```python
from build123d import *

# Parameters (mm, degrees)
F1_DEPTH  = 35
F2_R      = 30
F5_DEPTH  = 3
F8_DEPTH  = 3
F10_DEPTH = 2
F11_R     = 1.999


# Not quite as in the source:
# - a fillet or chamfer is up to 0.001 mm smaller than in the source, because OpenCascade refuses the exact size


with BuildPart() as f1:
    # F0 (on Right) → F1 (new body, symmetric)
    with BuildSketch(Plane.YZ):
        with BuildLine():
            Line((-75, 163), (-78, 163))
            Line((-78, 163), (-78, 8))
            ThreePointArc((-78, 8), (-75.6568542495, 2.3431457505), (-70, 0))
            Line((-70, 0), (0, 0))
            Line((0, 0), (0, 3))
            Line((0, 3), (-67, 3))
            ThreePointArc((-67, 3), (-72.6568542495, 5.3431457505), (-75, 11))
            Line((-75, 11), (-75, 163))
        make_face()
        with BuildLine():
            Line((0, 3), (0, 0))
            Line((0, 0), (70, 0))
            ThreePointArc((70, 0), (75.6568542495, 2.3431457505), (78, 8))
            Line((78, 8), (78, 163))
            Line((78, 163), (75, 163))
            Line((75, 163), (75, 11))
            ThreePointArc((75, 11), (72.6568542495, 5.3431457505), (67, 3))
            Line((67, 3), (0, 3))
        make_face()
    extrude(amount=F1_DEPTH, both=True)

    # F2
    f2_edges = [f1.edges().sort_by_distance(p)[0] for p in [
        (35, -76.5, 163),
        (35, 76.5, 163),
        (-35, 76.5, 163),
        (-35, -76.5, 163),
    ]]
    fillet(f2_edges, radius=F2_R)

    # F4 (on offset) → F5 (join)
    with BuildSketch(Plane(origin=(-35, 0, 0), x_dir=(0, -1, 0), z_dir=(-1, 0, 0))):
        with BuildLine():
            Line((-75, 133), (-78, 133))
            Line((-78, 133), (-78, 8))
            ThreePointArc((-78, 8), (-75.6568542495, 2.3431457505), (-70, 0))
            Line((-70, 0), (0, 0))
            Line((0, 0), (70, 0))
            ThreePointArc((70, 0), (75.6568542495, 2.3431457505), (78, 8))
            Line((78, 8), (78, 133))
            Line((78, 133), (75, 133))
            Line((75, 133), (0, 123))
            Line((0, 123), (-75, 133))
        make_face()
    extrude(amount=-F5_DEPTH)

    # F7 (on offset) → F8 (join)
    with BuildSketch(Plane.YZ.offset(35)):
        with BuildLine():
            Line((-78, 145), (-78, 8))
            ThreePointArc((-78, 8), (-75.6568542495, 2.3431457505), (-70, 0))
            Line((-70, 0), (0, 0))
            Line((0, 0), (70, 0))
            ThreePointArc((70, 0), (75.6568542495, 2.3431457505), (78, 8))
            Line((78, 8), (78, 145))
            Line((78, 145), (0, 145))
            Line((0, 145), (-78, 145))
        make_face()
    extrude(amount=-F8_DEPTH)

    # F9 (on offset) → F10 (join)
    with BuildSketch(Plane(origin=(-35, 0, 0), x_dir=(0, -1, 0), z_dir=(-1, 0, 0))):
        with BuildLine():
            add(Edge.make_bspline(
                [(22.5, 95), (22.5, 116.6506350946), (-11.25, 105.8253175473), (-45, 95), (-11.25, 84.1746824527), (22.5, 73.3493649054), (22.5, 95)],
                knots=[0, 0, 0, 2.0943951024, 2.0943951024, 4.1887902048, 4.1887902048, 6.2831853072, 6.2831853072, 6.2831853072], degree=2, weights=[1, 0.5, 1, 0.5, 1, 0.5, 1]))
        make_face()
    extrude(amount=F10_DEPTH)

    # F11 (radius 2 in the source; OpenCascade refuses exactly that, so slightly less here)
    f11_edges = [f1.edges().sort_by_distance(p)[0] for p in [
        (-37, 22.5, 95.000001),
    ]]
    fillet(f11_edges, radius=F11_R)


solid = f1.part
```
Can you work these out from the model? Positions are in its coordinate system, mm. A direction names the side the tool comes from. Coordinates: 2 decimals unless noted, no trailing zeros. Order: outer loops, then holes, each group sorted by start corner. A loop starts at its lowest first (then second) coordinate and runs counter-clockwise, first axis right, second up. Notation, with made-up numbers: (37, 52.25) -> (50, 52.25) arc R32 cw to (50, 90.25) -> close; hole circle Ø1 at (70.5, 87). An arc over 180 degrees is marked (long way). Write each question's results on one line, items separated by ' | '.
Item 1: I'm going to push flat-ended pins straight in: pin 1 Ø6 at (x, y) = (1, -48) entering from +Z; pin 2 Ø0.9 at (x, y) = (34, -11) entering from +Z. Where does each tip first touch, or does it pass through?
Results are:
pin 1: z = 3 | pin 2: z = 145
Item 2: I want a section at B-B, the plane y = -57. Write out the boundary of the cut face in (x, z).
Results are:
outline: (-35, 0) -> (35, 0) -> (35, 145) -> (32, 145) -> (32, 3) -> (-32, 3) -> (-32, 130.6) -> (-35, 130.6) -> close
Item 3: Which directions (+Z, -Z, +X, -X, +Y, -Y) give clear straight access to the entire face, cutting with the end or side of a thin tool? Please do faces 5 (the face through (-32, 1, 69)), 6 (the face through (-33.52, -38.02, 128.07)), 7 (the face through (21.23, 76.48, 158.23)).
Results are:
face 5: +Z | face 6: +Z, -X | face 7: +Z, +X, +Y, -Y
Item 4: If I drill on line 1 along X through (y, z) = (-27.5, 76); line 2 along Y through (x, z) = (-8, 67); line 3 along Z through (x, y) = (-26.5, 45.5), over which ranges is the centre line in solid material (lowest first)?
Results are:
line 1: -35 to -32, 32 to 35 | line 2: -78 to -75, 75 to 78 | line 3: 0 to 3
Item 5: I want a section at C-C, the plane z = 128.5. Write out the boundary of the cut face in (x, y).
Results are:
outline: (-35, -78) -> (35, -78) -> (35, 78) -> (-35, 78) -> (-35, 41.25) -> (-32, 41.25) -> (-32, 75) -> (32, 75) -> (32, -75) -> (-32, -75) -> (-32, -41.25) -> (-35, -41.25) -> close
Item 6: If we mould it in two halves opening along X, with no side actions, what happens to faces 1 (the face through (0.49, 75.594, 2.281)), 2 (the face through (32, -1, 75)), 3 (the face through (0.448, -72.594, 5.281)), 4 (the face through (-35, -1, 67))? For each: +X half, -X half, draft (parallel to the pull), parting line (faces both ways), or undercut.
Results are:
face 1: draft | face 2: undercut | face 3: undercut | face 4: -X half
Item 7: I want a section at A-A, the plane z = 60.5. Write out the boundary of the cut face in (x, y), then the cut area to 3 significant figures.
Results are:
outline: (-35, -78) -> (35, -78) -> (35, 78) -> (-35, 78) -> close; hole (-32, -75) -> (32, -75) -> (32, 75) -> (-32, 75) -> close | area: 1,320 mm²
Item 8: I want a section at D-D, the plane x = -27.5. Write out the boundary of the cut face in (y, z), then the cut area to 3 significant figures.
Results are:
outline: (-78, 8) arc R8 ccw to (-70, 0) -> (70, 0) arc R8 ccw to (78, 8) -> (78, 152.84) -> (75, 152.84) -> (75, 11) arc R8 cw to (67, 3) -> (-67, 3) arc R8 cw to (-75, 11) -> (-75, 152.84) -> (-78, 152.84) -> close | area: 1,370 mm²
